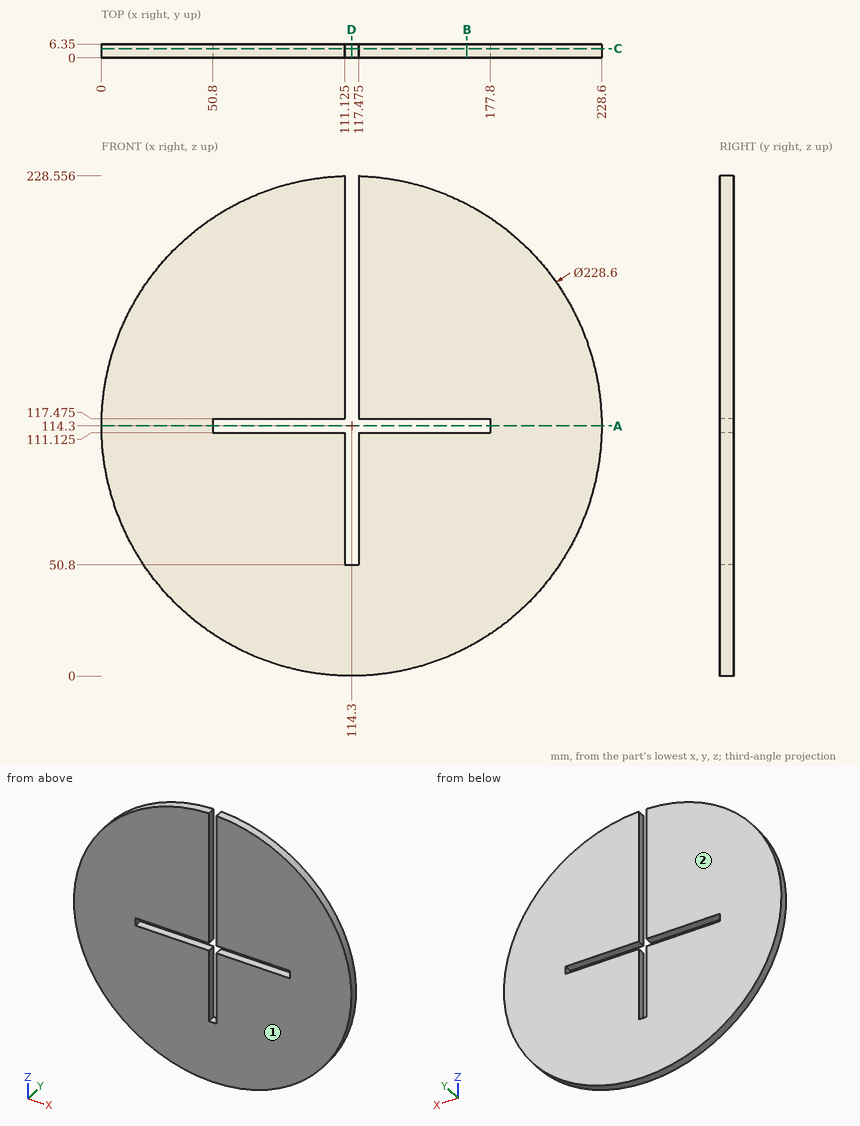
Geometry: see drawing. Coordinates: mm, zero at the bounding-box minimum. Give positions to 0.01 mm unless a question says otherwise; leave off trailing zeros. Write each loop counter-clockwise with the first axis right and the second up, starting at its lowest first coordinate (ties: lowest second). Pieces come first, ordered by that corner, then holes. Notation, with made-up numbers: M 52.25,35 L 81.25,35 A10 cw 81.25,53 Z; hole C 75.25,49 d5. An arc over 180 degrees is marked long. Answer as a JSON object with one key per item and string values.
Q1. Cut plane D-D, the plane x = 114.3. Return the cut outline in (y, z).
Geometry check:
{"outline": "M 0,0 L 6.35,0 L 6.35,50.8 L 0,50.8 Z"}
Q2. Ray query, line 1 along X through (y, z) = (3.25, 184) (1 decimal); line 2 along Z through (x, y) = (150, 2.25) (1 decimal); line 3 along Z through (x, y) = (146.5, 6) (1 decimal). Return the intervals inside material, ascending.
Geometry check:
{"line 1": "x = 23.7 to 111.1, 117.5 to 204.9", "line 2": "z = 5.7 to 111.1, 117.5 to 222.9", "line 3": "z = 4.6 to 111.1, 117.5 to 224"}
Q3. Cut plane A-A, the plane z = 114.3. Return the cut outline in (x, y), then the cut area to 3 significant figures.
Geometry check:
{"outline": "M 0,0 L 50.8,0 L 50.8,6.35 L 0,6.35 Z; M 177.8,0 L 228.6,0 L 228.6,6.35 L 177.8,6.35 Z", "area": "645 mm^2"}
Q4. Mould query, pull axis Y, two halves, no side actions, for the marked faces 1 and 2. Classes: +Y half, -Y half, draft (parallel to the pull), parting line (faces both ways), or undercut.
Geometry check:
{"face 1": "-Y half", "face 2": "+Y half"}
Q5. Cut plane C-C, the plane y = 4.25. Return the cut outline in (x, z) (3 decimals), then the cut area to 3 significant figures.
Geometry check:
{"outline": "M 50.8,111.125 L 50.8,117.475 L 111.125,117.475 L 111.125,228.556 A114.3 ccw long 117.475,228.556 L 117.475,117.475 L 177.8,117.475 L 177.8,111.125 L 117.475,111.125 L 117.475,50.8 L 111.125,50.8 L 111.125,111.125 Z", "area": "39,100 mm^2"}
Q6. Cut plane B-B, the plane x = 167. Return the cut outline in (y, z) (3 decimals), then the cut area to 3 significant figures.
Geometry check:
{"outline": "M 0,12.874 L 6.35,12.874 L 6.35,111.125 L 0,111.125 Z; M 0,117.475 L 6.35,117.475 L 6.35,215.726 L 0,215.726 Z", "area": "1,250 mm^2"}
Q7. Contact query for flat-ended pins moving along their axis: P1, Ø3, axis at x = 83, y = 4.5, coming from the -Z side; P2, Ø3, axis at x = 115, y = 3.5, coming from the +Z side; P3, Ø6, axis at x = 174, z = 50.5, coming from the -Y side; P4, Ø1.9, axis at y = 3, z = 175, coming from the -X side. Output: stop coordinate, or through.
Geometry check:
{"P1": "stops at z = 3.95", "P2": "stops at z = 50.8", "P3": "stops at y = 0", "P4": "stops at x = 16.86"}
